The drawing under review shows one solid part. Ordinate dimensions are in mm from its lowest x, y, z. A direction names the side the tool comes from. Give positions to 0.01 mm unless a question says otherwise; leave off trailing zeros. Order: outer loops, then holes, each group sorted by start corner. A loop starts at its lowest first (then second) coordinate and runs counter-clockwise, first axis right, second up. Notation, with made-up numbers: (-15.5, 43.25) -> (14.5, 43.25) arc R20 ccw to (14.5, 79.25) -> close; hole circle Ø9 at (-30.5, -7.5). An arc over 180 degrees is marked (long way). Return JSON: item names as keys, results as strings. Group by question number.
1) To check wall thickness, follow line 1 along X through (y, z) = (2.5, 13.25); line 2 along Z through (x, y) = (5.5, 2.5). State the ranges of each line that lie inside material, in increasing order.
2) For the marked faces 5, 6 and 7, list the 3-axis set-ups (+Z, -Z, +X, -X, +Y, -Y) from which the entire face can be reached by the end or side of a thin tool; tool diameter is ignored.
3) Insertion check: P1, Ø6.5, axis at x = 11.5, y = 9.5, coming from the +Z side; P2, Ø4, axis at x = 9, y = 8.5, coming from the -Z side; P3, Ø1.6, axis at y = 3.5, z = 8.5, coming from the +X side. Each pin has a flat end and moves straight along its axis. Give the tip position at first contact, or say it passes through.
4) The part is to be moulded in two halves that separate along X. For the marked faces 1, 2, 3 and 4, say which applies: released by +X, released by -X, zero draft, split by the parting line, or undercut.
5) Add section A-A (x = 7). Give the boundary of the cut face in (y, z).
6) Add section C-C (y = 7). Give the boundary of the cut face in (x, z).
7) Add section D-D (x = 3). Give the boundary of the cut face in (y, z), then the cut area to 3 significant figures.
8) Add section B-B (z = 10.5). Give the boundary of the cut face in (x, y).
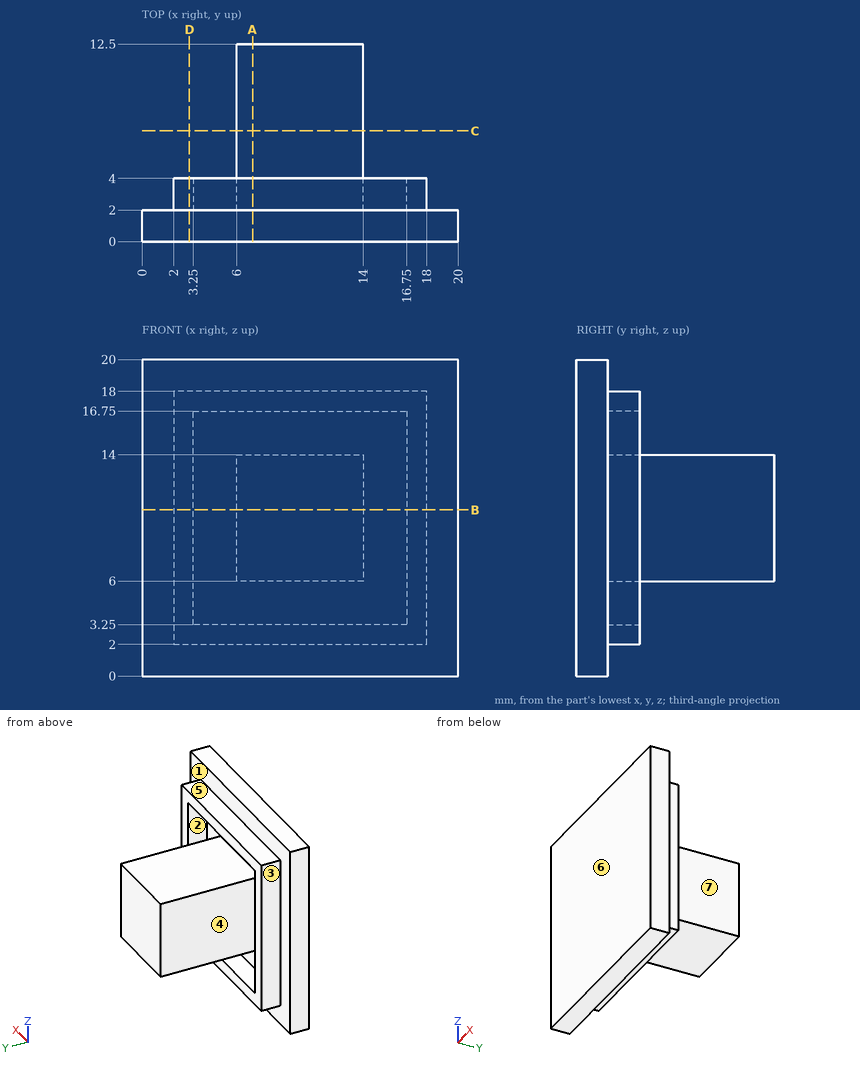
Evaluation:
{
 "1": {"line 1": "2 to 3.25, 6 to 14, 16.75 to 18", "line 2": "2 to 3.25, 16.75 to 18"},
 "2": {"face 5": "+Z, +X, -X, +Y", "face 6": "+Z, -Z, +X, -X, -Y", "face 7": "+Y"},
 "3": {"P1": "z = 14", "P2": "z = 6", "P3": "x = 18"},
 "4": {"face 1": "zero draft", "face 2": "undercut", "face 3": "released by -X", "face 4": "undercut"},
 "5": {"outline": "(0, 0) -> (2, 0) -> (2, 2) -> (4, 2) -> (4, 3.25) -> (2, 3.25) -> (2, 6) -> (12.5, 6) -> (12.5, 14) -> (2, 14) -> (2, 16.75) -> (4, 16.75) -> (4, 18) -> (2, 18) -> (2, 20) -> (0, 20) -> close"},
 "6": {"outline": "(6, 6) -> (14, 6) -> (14, 14) -> (6, 14) -> close"},
 "7": {"outline": "(0, 0) -> (2, 0) -> (2, 2) -> (4, 2) -> (4, 18) -> (2, 18) -> (2, 20) -> (0, 20) -> close", "area": "72.0 mm^2"},
 "8": {"outline": "(0, 0) -> (20, 0) -> (20, 2) -> (18, 2) -> (18, 4) -> (16.75, 4) -> (16.75, 2) -> (14, 2) -> (14, 12.5) -> (6, 12.5) -> (6, 2) -> (3.25, 2) -> (3.25, 4) -> (2, 4) -> (2, 2) -> (0, 2) -> close"}
}
